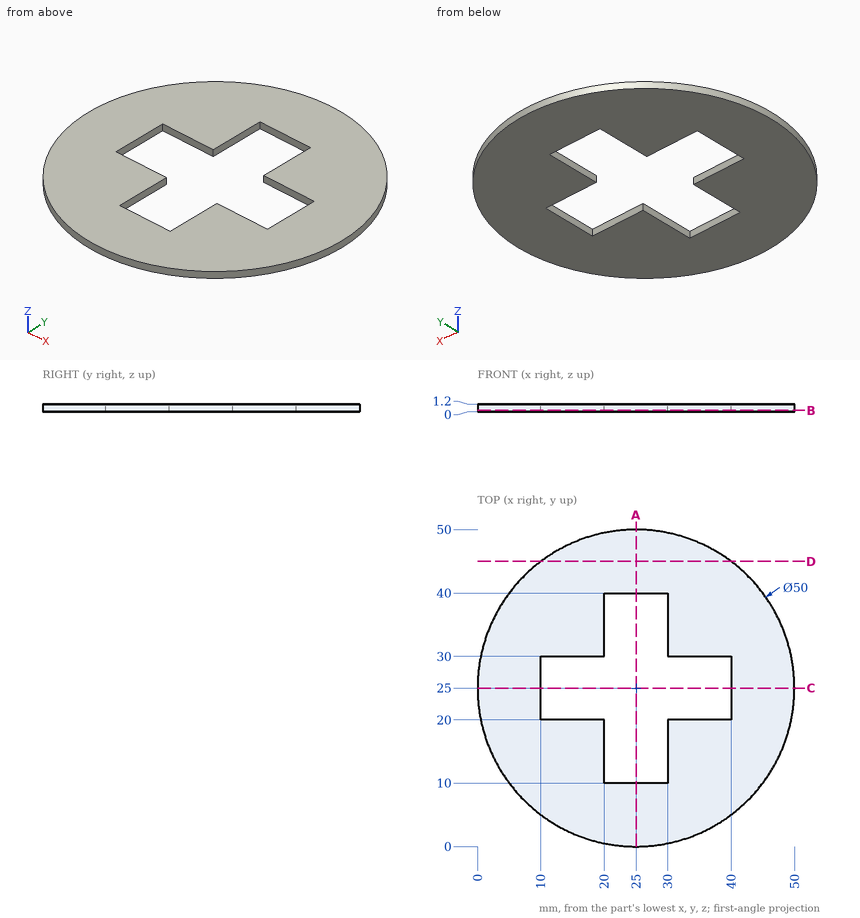
Source: three-view drawing plus pictorial views. Frame: mm from the lowest corner of the part. Coordinates: 2 decimals unless noted, no trailing zeros. Order: outer loops, then holes, each group sorted by start corner. A loop starts at its lowest first (then second) coordinate and runs counter-clockwise, first axis right, second up. Notation, with made-up numbers: M 39,2.5 L 58,2.5 A20 ccw 58,41.5 Z; hole C -16.75,58.25 d11. An arc over 180 degrees is marked long. One line per question, with ' | ' between items.
Item 1: Pin query (flat end, axial travel): pin 1 (1.5 mm diameter, centred on x = 8, y = 6.5, fed in from +Z); pin 2 (0.6 mm diameter, centred on y = 17.5, z = 0.5, fed in from +X); pin 3 (0.6 mm diameter, centred on y = 35.5, z = 1, fed in from -X); pin 4 (0.6 mm diameter, centred on x = 16, z = 0.5, fed in from -Y). Return the tip coordinate at first contact, or that it passes through.
Geometry results:
pin 1: stops at z = 1.2 | pin 2: stops at x = 48.94 | pin 3: stops at x = 2.18 | pin 4: stops at y = 1.56
Item 2: Section A-A (x = 25). Output: boundary loops of the cut face in (y, z), then the cut area to 3 significant figures.
Geometry results:
outline: M 0,0 L 10,0 L 10,1.2 L 0,1.2 Z; M 40,0 L 50,0 L 50,1.2 L 40,1.2 Z | area: 24.0 mm^2
Item 3: Ray query, line 1 along Y through (x, z) = (11.5, 1.1); line 2 along X through (y, z) = (36, 1); line 3 along X through (y, z) = (12.5, 0.6). Return the intervals inside material, ascending.
Geometry results:
line 1: y = 3.96 to 20, 30 to 46.04 | line 2: x = 2.55 to 20, 30 to 47.45 | line 3: x = 3.35 to 20, 30 to 46.65
Item 4: Section D-D (y = 45). Output: boundary loops of the cut face in (x, z), then the cut area to 3 significant figures.
Geometry results:
outline: M 10,0 L 40,0 L 40,1.2 L 10,1.2 Z | area: 36.0 mm^2
Item 5: Section B-B (z = 0.2). Output: boundary loops of the cut face in (x, y).
Geometry results:
outline: C 25,25 d50; hole M 10,20 L 20,20 L 20,10 L 30,10 L 30,20 L 40,20 L 40,30 L 30,30 L 30,40 L 20,40 L 20,30 L 10,30 Z
